The listing builds one solid part. Answer for the finished solid, in the listing's coordinates (mm). Give positions to 0.01 mm unless a question says otherwise; leave off trailing zeros. Order: outer loops, then holes, each group sorted by start corner. A loop starts at its lowest first (then second) coordinate and runs counter-clockwise, first axis right, second up. Notation, with made-up numbers: (59, -21) - (88, -21) arc R16 ccw to (88, -8) - close; hole circle Ø2 at (13, -16). An arc over 180 degrees is marked (long way). Answer in a Markdown table with one row per item.
from build123d import *

# Parameters (mm, degrees)
ESQUISSE1_R                  = 3
BOSS_EXTRU_1_DEPTH           = 94
ENL_V_MAT_EXTRU_1_DEPTH      = 95.09569597
ENL_V_MAT_EXTRU_1_DEPTH_BACK = 95.09569597
ESQUISSE2_R                  = 1.25
CHANFREIN1_SIZE              = 0.3


with BuildPart() as part:
    # Esquisse1 → Boss.-Extru.1 (new body)
    with BuildSketch(Plane.XY):
        Circle(ESQUISSE1_R)
    extrude(amount=BOSS_EXTRU_1_DEPTH)

    # Esquisse2 → Enlèv. mat.-Extru.1 (cut, two sides: drawn at the far end of the back side and taken through both)
    with BuildSketch(Plane(origin=(0, 0, 0), x_dir=(1, 0, 0), z_dir=(0, 1, 0)).offset(-ENL_V_MAT_EXTRU_1_DEPTH_BACK)):
        with Locations(Location((0, -9, 0), (0, 0, 270))):
            Circle(ESQUISSE2_R)
    extrude(amount=ENL_V_MAT_EXTRU_1_DEPTH + ENL_V_MAT_EXTRU_1_DEPTH_BACK, mode=Mode.SUBTRACT)

    # Chanfrein1
    chanfrein1_edges = [part.edges().sort_by_distance(p)[0] for p in [
        (-3, 0, 0),
        (-3, 0, 94),
    ]]
    chamfer(chanfrein1_edges, length=CHANFREIN1_SIZE)


solid = part.part
Item 1: Find section A-A on x = 0. Write down the section's boundary in (y, z).
Answer block:
| item | result |
|---|---|
| outline | (-3, 0.3) - (-2.7, 0) - (2.7, 0) - (3, 0.3) - (3, 7.75) - (-3, 7.75) - close; (-3, 10.25) - (3, 10.25) - (3, 93.7) - (2.7, 94) - (-2.7, 94) - (-3, 93.7) - close |
Item 2: Each of these flat-tipped pins is pushed along its axis until it touches: P1, Ø2, axis at x = -1.5, z = 48, coming from the -Y side; P2, Ø1.5, axis at y = -2, z = 10.5, coming from the -X side; P3, Ø2, axis at x = -1.5, z = 59, coming from the +Y side. Where does it stop, or does it pass through?
Answer block:
| item | result |
|---|---|
| P1 | y = -2.96 |
| P2 | x = -2.73 |
| P3 | y = 2.96 |
Item 3: Determine the mould class of faces 1 (the face through (0, 0, 94)), 2 (the face through (0, 0, 0)), 3 (the face through (-3, 0, 46)), 4 (the face through (0.05, -0.04, 7.75)) for opening direction Z: pulls with the +Z half, pulls with the -Z half, needs draft (parallel to the pull), parting line crosses it, or undercut.
Answer block:
| item | result |
|---|---|
| face 1 | pulls with the +Z half |
| face 2 | pulls with the -Z half |
| face 3 | needs draft |
| face 4 | undercut |
Item 4: Find section C-C on z = 9. Write down the section's boundary in (x, y).
Answer block:
| item | result |
|---|---|
| outline | (-1.25, -2.73) - (-1.25, 2.73) arc R3 ccw to start; (1.25, -2.73) arc R3 ccw to (1.25, 2.73) - close |
Item 5: Consider line 1 (Z direction, x = 0, y = 0.25); line 2 (Z direction, x = -0.75, y = -0.5); line 3 (X direction, y = 1.5, z = 9). Determine where each line is inside the solid, lowest interval first.
Answer block:
| item | result |
|---|---|
| line 1 | 0 to 7.75, 10.25 to 94 |
| line 2 | 0 to 8, 10 to 94 |
| line 3 | -2.6 to -1.25, 1.25 to 2.6 |
Item 6: Find section B-B on z = 85. Write down the section's boundary in (x, y), then the cut area to 3 significant figures.
Answer block:
| item | result |
|---|---|
| outline | circle Ø6 at (0, 0) |
| area | 28.3 mm² |
